Here's how the part is built. I have some questions about the finished solid (model axes, mm). Face numbers are marked on the shaded views. A direction names the side the tool comes from. Coordinates: 2 decimals unless noted, no trailing zeros. Write each loop counter-clockwise with the first axis right and the second up, starting at its lowest first coordinate (ties: lowest second). Pieces come first, ordered by that corner, then holes.
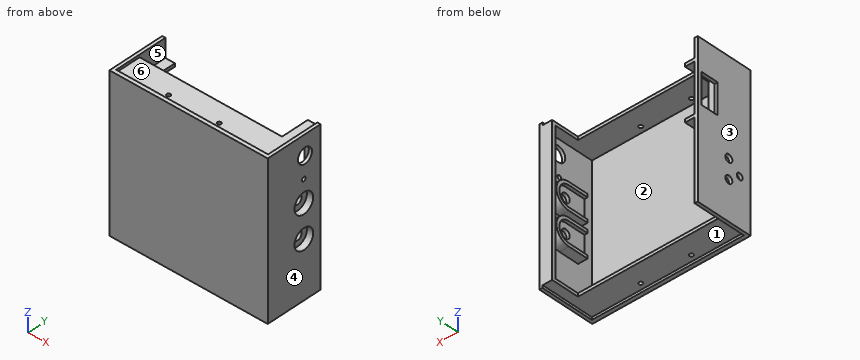
```python
from build123d import *

# Parameters (mm, degrees)
SKETCH2_W                = 125
SKETCH2_H                = 120.1
BOSS_EXTRUDE1_DEPTH      = 45
SKETCH3_W                = 120
SKETCH3_H                = 111.1
CUT_EXTRUDE1_DEPTH       = 39
SKETCH4_W                = 120
SKETCH4_H                = 2
CUT_EXTRUDE3_DEPTH       = 43
LPATTERN1_COUNT          = 2
LPATTERN1_PITCH          = 118.1
SKETCH9_W                = 112.5
SKETCH9_H                = 116.1
CUT_EXTRUDE6_DEPTH       = 23
SKETCH11_R               = 3
CUT_EXTRUDE7_DEPTH       = 3.5
SKETCH15_R               = 2.5
CUT_EXTRUDE9_DEPTH       = 3.5
SKETCH13_W               = 24
SKETCH13_H               = 14
CUT_EXTRUDE10_DEPTH      = 3.5
BOSS_EXTRUDE3_DEPTH      = 7.5
BOSS_EXTRUDE4_DEPTH      = 10
LPATTERN3_COUNT          = 2
LPATTERN3_PITCH          = 26
SKETCH22_R               = 3.5
CUT_EXTRUDE11_DEPTH      = 10
LPATTERN4_COUNT          = 2
LPATTERN4_PITCH          = 26
SKETCH23_R               = 1.6
CUT_EXTRUDE12_DEPTH      = 10
SKETCH26_R               = 3.5
BOSS_EXTRUDE10_DEPTH     = 7.5
LPATTERN9_COUNT          = 2
LPATTERN9_PITCH          = 26
SKETCH27_R               = 6
CUT_EXTRUDE13_DEPTH      = 7.5
SKETCH28_R               = 1.5
CUT_EXTRUDE14_DEPTH      = 61.05
CUT_EXTRUDE14_DEPTH_BACK = 61.05
SKETCH30_R               = 8
CUT_EXTRUDE15_DEPTH      = 5
LPATTERN10_COUNT         = 2
LPATTERN10_PITCH         = 26


with BuildPart() as part:
    # Sketch2 → Boss-Extrude1 (new body)
    with BuildSketch(Plane(origin=(0, 0, 0), x_dir=(1, 0, 0), z_dir=(0, 1, 0))):
        Rectangle(SKETCH2_W, SKETCH2_H)
    extrude(amount=BOSS_EXTRUDE1_DEPTH)

    # Sketch3 → Cut-Extrude1 (cut)
    with BuildSketch(Plane(origin=(0, 3, 0), x_dir=(1, 0, 0), z_dir=(0, 1, 0))):
        Rectangle(SKETCH3_W, SKETCH3_H)
    extrude(amount=CUT_EXTRUDE1_DEPTH, mode=Mode.SUBTRACT)

    # Sketch4 → Cut-Extrude3 (cut, through all)
    with BuildSketch(Plane(origin=(0, 3, 0), x_dir=(1, 0, 0), z_dir=(0, 1, 0))):
        with Locations((0, -59.05)):
            Rectangle(SKETCH4_W, SKETCH4_H)
    cut_extrude3 = extrude(amount=CUT_EXTRUDE3_DEPTH, mode=Mode.SUBTRACT)

    # LPattern1: Cut-Extrude3 ×2
    with Locations(*[(0, 0, -i * LPATTERN1_PITCH) for i in range(1, LPATTERN1_COUNT)]):
        add(cut_extrude3, mode=Mode.SUBTRACT)

    # Sketch9 → Cut-Extrude6 (cut, through all)
    with BuildSketch(Plane(origin=(0, 23, 0), x_dir=(1, 0, 0), z_dir=(0, 1, 0))):
        with Locations((-3.75, 0)):
            Rectangle(SKETCH9_W, SKETCH9_H)
    extrude(amount=CUT_EXTRUDE6_DEPTH, mode=Mode.SUBTRACT)

    # Sketch11 → Cut-Extrude7 (cut, through all)
    with BuildSketch(Plane(origin=(-60, 0, 0), x_dir=(0, 0, -1), z_dir=(1, 0, 0))):
        with Locations((29.45, 18.51)):
            Circle(SKETCH11_R)
        with Locations((14.05, 18.51)):
            Circle(SKETCH11_R)
    extrude(amount=-CUT_EXTRUDE7_DEPTH, mode=Mode.SUBTRACT)

    # Sketch15 → Cut-Extrude9 (cut, through all)
    with BuildSketch(Plane(origin=(-60, 0, 0), x_dir=(0, 0, -1), z_dir=(1, 0, 0))):
        with Locations((22.117427494, 9.198406991)):
            Circle(SKETCH15_R)
    extrude(amount=-CUT_EXTRUDE9_DEPTH, mode=Mode.SUBTRACT)

    # Sketch13 → Cut-Extrude10 (cut, through all)
    with BuildSketch(Plane(origin=(-60, 0, 0), x_dir=(0, 0, -1), z_dir=(1, 0, 0))):
        with Locations((-23.885447562, 35)):
            Rectangle(SKETCH13_W, SKETCH13_H)
    extrude(amount=-CUT_EXTRUDE10_DEPTH, mode=Mode.SUBTRACT)

    # Sketch17 → Boss-Extrude3 (add)
    with BuildSketch(Plane(origin=(-60, 0, 0), x_dir=(0, 0, -1), z_dir=(1, 0, 0))):
        Polygon((-42.885447562, 45), (-42.885447562, 25), (-4.885447562, 25), (-4.885447562, 45), (-2.385447562, 45), (-2.385447562, 22.5), (-45.385447562, 22.5), (-45.385447562, 45), align=None)
    extrude(amount=BOSS_EXTRUDE3_DEPTH)

    # Sketch18 → Boss-Extrude4 (add)
    with BuildSketch(Plane(origin=(62.5, 0, 0), x_dir=(0, 0, -1), z_dir=(1, 0, 0))):
        with BuildLine():
            Line((7.45, 30.801411804), (7.45, 14.801411804))
            Line((7.45, 14.801411804), (4.95, 14.801411804))
            Line((4.95, 14.801411804), (4.95, 30.801411804))
            ThreePointArc((4.95, 30.801411804), (15.45, 41.301411804), (25.95, 30.801411804))
            Line((25.95, 30.801411804), (25.95, 14.801411804))
            Line((25.95, 14.801411804), (23.45, 14.801411804))
            Line((23.45, 14.801411804), (23.45, 30.801411804))
            ThreePointArc((23.45, 30.801411804), (15.45, 38.801411804), (7.45, 30.801411804))
        make_face()
    boss_extrude4 = extrude(amount=-BOSS_EXTRUDE4_DEPTH)

    # LPattern3: Boss-Extrude4 ×2
    with Locations(*[(0, 0, i * LPATTERN3_PITCH) for i in range(1, LPATTERN3_COUNT)]):
        add(boss_extrude4)

    # Sketch22 → Cut-Extrude11 (cut)
    with BuildSketch(Plane(origin=(62.5, 0, 0), x_dir=(0, 0, -1), z_dir=(1, 0, 0))):
        with Locations((15.45, 30.801411804)):
            Circle(SKETCH22_R)
    cut_extrude11 = extrude(amount=-CUT_EXTRUDE11_DEPTH, mode=Mode.SUBTRACT)

    # LPattern4: Cut-Extrude11 ×2
    with Locations(*[(0, 0, i * LPATTERN4_PITCH) for i in range(1, LPATTERN4_COUNT)]):
        add(cut_extrude11, mode=Mode.SUBTRACT)

    # Sketch23 → Cut-Extrude12 (cut)
    with BuildSketch(Plane(origin=(62.5, 0, 0), x_dir=(0, 0, -1), z_dir=(1, 0, 0))):
        with Locations((-28.05, 30.801411804)):
            Circle(SKETCH23_R)
    extrude(amount=-CUT_EXTRUDE12_DEPTH, mode=Mode.SUBTRACT)

    # Sketch26 → Boss-Extrude10 (add)
    with BuildSketch(Plane(origin=(62.5, 0, 0), x_dir=(0, 0, -1), z_dir=(1, 0, 0))):
        with BuildLine():
            Line((23.45, 14.801411804), (7.45, 14.801411804))
            Line((7.45, 14.801411804), (7.45, 30.801411804))
            ThreePointArc((7.45, 30.801411804), (15.45, 38.801411804), (23.45, 30.801411804))
            Line((23.45, 30.801411804), (23.45, 14.801411804))
        make_face()
        with Locations((15.45, 30.801411804)):
            Circle(SKETCH26_R, mode=Mode.SUBTRACT)
    boss_extrude10 = extrude(amount=-BOSS_EXTRUDE10_DEPTH)

    # LPattern9: Boss-Extrude10 ×2
    with Locations(*[(0, 0, i * LPATTERN9_PITCH) for i in range(1, LPATTERN9_COUNT)]):
        add(boss_extrude10)

    # Sketch27 → Cut-Extrude13 (cut)
    with BuildSketch(Plane(origin=(62.5, 0, 0), x_dir=(0, 0, -1), z_dir=(1, 0, 0))):
        with Locations((-44.552239633, 31.709599536)):
            Circle(SKETCH27_R)
    extrude(amount=-CUT_EXTRUDE13_DEPTH, mode=Mode.SUBTRACT)

    # Sketch28 → Cut-Extrude14 (cut, two sides)
    with BuildSketch(Plane.XY) as cut_extrude14_sk:
        with Locations((-23, 7.75)):
            Circle(SKETCH28_R)
        with Locations((17, 7.75)):
            Circle(SKETCH28_R)
    extrude(amount=CUT_EXTRUDE14_DEPTH, mode=Mode.SUBTRACT)
    extrude(cut_extrude14_sk.sketch, amount=-CUT_EXTRUDE14_DEPTH_BACK, mode=Mode.SUBTRACT)

    # Sketch30 → Cut-Extrude15 (cut)
    with BuildSketch(Plane(origin=(62.5, 0, 0), x_dir=(0, 0, -1), z_dir=(1, 0, 0))):
        with Locations((15.45, 30.801411804)):
            Circle(SKETCH30_R)
    cut_extrude15 = extrude(amount=-CUT_EXTRUDE15_DEPTH, mode=Mode.SUBTRACT)

    # LPattern10: Cut-Extrude15 ×2
    with Locations(*[(0, 0, i * LPATTERN10_PITCH) for i in range(1, LPATTERN10_COUNT)]):
        add(cut_extrude15, mode=Mode.SUBTRACT)


solid = part.part
```
1) I need wall thicknesses on probe 1 along Y at (x, z) = (59.5, 10.55); probe 2 along Y at (x, z) = (56.85, -15.45); probe 3 along Y at (x, z) = (-62, -14). Which ranges of each line are inside material? Lowest first, please.
Values follow:
probe 1: y = 0 to 3, 14.8 to 22.8, 38.8 to 41.3, 42 to 45
probe 2: y = 0 to 3, 14.8 to 27.3, 34.3 to 41.3, 42 to 45
probe 3: y = 0 to 15.51, 21.51 to 45
2) Will these pins go through, and if not, where does the flat tip stop? pin 1 (4 mm diameter, centred on x = 41.5, y = 14.5, fed in from +Z); pin 2 (21 mm diameter, centred on x = -10.5, y = 22, fed in from -Z); pin 3 (1.6 mm diameter, centred on x = -21.5, z = 59.5, fed in from +Y).
Values follow:
pin 1: stops at z = 58.05
pin 2: stops at z = -58.05
pin 3: stops at y = 3
3) Imagine slicing it at D-D on z = 8.5. Please give me the cut outline in (x, y), then the cut area to 3 significant figures.
Values follow:
outline: (-62.5, 0) - (62.5, 0) - (62.5, 23.07) - (57.5, 23.07) - (57.5, 27.96) - (55, 27.96) - (55, 14.8) - (60, 14.8) - (60, 3) - (-60, 3) - (-60, 22.5) - (-52.5, 22.5) - (-52.5, 25) - (-60, 25) - (-60, 45) - (-62.5, 45) - close; (52.5, 38.53) - (55, 38.53) - (55, 33.64) - (57.5, 33.64) - (57.5, 38.53) - (62.5, 38.53) - (62.5, 45) - (52.5, 45) - (52.5, 42) - (60, 42) - (60, 41.1) - (52.5, 41.1) - close
area: 673 mm2
4) Imagine slicing it at A-A on x = -23. Please give me the cut outline in (y, z), then the cut area to 3 significant figures.
Values follow:
outline: (0, -60.05) - (3, -60.05) - (3, -58.05) - (6.25, -58.05) - (6.25, -55.55) - (3, -55.55) - (3, 55.55) - (6.25, 55.55) - (6.25, 58.05) - (3, 58.05) - (3, 60.05) - (0, 60.05) - close; (9.25, -58.05) - (23, -58.05) - (23, -55.55) - (9.25, -55.55) - close; (9.25, 55.55) - (23, 55.55) - (23, 58.05) - (9.25, 58.05) - close
area: 445 mm2
5) We'd pull the mould along Z, two halves only. Please class the marked faces 1, 2 and 3: pulls with the +Z half, pulls with the -Z half, needs draft (parallel to the pull), parting line crosses it, or undercut.
Values follow:
face 1: pulls with the -Z half
face 2: undercut
face 3: needs draft
6) Imagine slicing it at C-C on z = -15.45. Please give me the cut outline in (x, y).
Values follow:
outline: (-62.5, 0) - (62.5, 0) - (62.5, 22.8) - (57.5, 22.8) - (57.5, 27.3) - (55, 27.3) - (55, 14.8) - (60, 14.8) - (60, 3) - (-60, 3) - (-60, 15.86) - (-62.5, 15.86) - close; (-62.5, 21.16) - (-60, 21.16) - (-60, 45) - (-62.5, 45) - close; (52.5, 38.8) - (55, 38.8) - (55, 34.3) - (57.5, 34.3) - (57.5, 38.8) - (62.5, 38.8) - (62.5, 45) - (52.5, 45) - (52.5, 42) - (60, 42) - (60, 41.3) - (52.5, 41.3) - close
7) On a 3-axis mill with a long thin cutter (end or side, diameter ignored), from which of +Z, -Z, +X, -X, +Y, -Y can I reach the whole of each face in a straight line? I mean the marked faces 4, 5 and 6. Say none if no direction works.
Values follow:
face 4: +Z, -Z, +X, +Y, -Y
face 5: none
face 6: +Z, +Y
8) Imagine slicing it at B-B on z = -29.45. Please give me the cut outline in (x, y).
Values follow:
outline: (-62.5, 0) - (62.5, 0) - (62.5, 45) - (52.5, 45) - (52.5, 42) - (60, 42) - (60, 3) - (-60, 3) - (-60, 15.51) - (-62.5, 15.51) - close; (-62.5, 21.51) - (-60, 21.51) - (-60, 45) - (-62.5, 45) - close
